from build123d import *

# Parameters (mm, degrees)
SKETCH1_W           = 70
SKETCH1_H           = 170
BOSS_EXTRUDE1_DEPTH = 5
SKETCH2_W           = 70
SKETCH2_H           = 5
BOSS_EXTRUDE2_DEPTH = 25
SKETCH3_W           = 70
SKETCH3_H           = 5
BOSS_EXTRUDE3_DEPTH = 50
SKETCH4_W           = 3
SKETCH4_H           = 15
BOSS_EXTRUDE4_DEPTH = 20
CUT_EXTRUDE1_REACH  = 98.695
SKETCH6_R           = 12.5
SKETCH6_R_2         = 7
SKETCH6_R_3         = 8.5
SKETCH6_R_4         = 8
SKETCH6_R_5         = 4.5
SKETCH6_R_6         = 3
SKETCH7_R           = 4.797792648
SKETCH7_R_2         = 3.987535838
SKETCH7_W           = 10.549301712
SKETCH7_H           = 5.014130384
BOSS_EXTRUDE5_DEPTH = 3


with BuildPart() as part:
    # Sketch1 → Boss-Extrude1 (new body)
    with BuildSketch(Plane.XY):
        Rectangle(SKETCH1_W, SKETCH1_H)
    extrude(amount=BOSS_EXTRUDE1_DEPTH)

    # Sketch2 → Boss-Extrude2 (add)
    with BuildSketch(Plane.XY.offset(5)):
        with Locations((0, -82.5)):
            Rectangle(SKETCH2_W, SKETCH2_H)
    extrude(amount=BOSS_EXTRUDE2_DEPTH)

    # Sketch3 → Boss-Extrude3 (add)
    with BuildSketch(Plane(origin=(0, -80, 0), x_dir=(1, 0, 0), z_dir=(0, 1, 0))):
        with Locations((0, -27.5)):
            Rectangle(SKETCH3_W, SKETCH3_H)
    extrude(amount=BOSS_EXTRUDE3_DEPTH)

    # Sketch4 → Boss-Extrude4 (add)
    with BuildSketch(Plane.XY.offset(5)):
        with Locations((-33.5, -37.5)):
            Rectangle(SKETCH4_W, SKETCH4_H)
        with Locations((33.5, -37.5)):
            Rectangle(SKETCH4_W, SKETCH4_H)
    extrude(amount=BOSS_EXTRUDE4_DEPTH)

    # Sketch6 → Cut-Extrude1 (cut, up to next)
    with BuildSketch(Plane.XY.offset(30), mode=Mode.PRIVATE) as cut_extrude1_sk1:
        with Locations((0, -45)):
            Circle(SKETCH6_R)
    cut_extrude1_tool1 = extrude(cut_extrude1_sk1.sketch, amount=-CUT_EXTRUDE1_REACH, mode=Mode.PRIVATE) & part.part
    # Sketch6 → Cut-Extrude1 (cut, up to next)
    with BuildSketch(Plane.XY.offset(30), mode=Mode.PRIVATE) as cut_extrude1_sk2:
        with Locations((-25, -40)):
            Circle(SKETCH6_R_2)
    cut_extrude1_tool2 = extrude(cut_extrude1_sk2.sketch, amount=-CUT_EXTRUDE1_REACH, mode=Mode.PRIVATE) & part.part
    # Sketch6 → Cut-Extrude1 (cut, up to next)
    with BuildSketch(Plane.XY.offset(30), mode=Mode.PRIVATE) as cut_extrude1_sk3:
        with Locations((25, -40)):
            Circle(SKETCH6_R_2)
    cut_extrude1_tool3 = extrude(cut_extrude1_sk3.sketch, amount=-CUT_EXTRUDE1_REACH, mode=Mode.PRIVATE) & part.part
    # Sketch6 → Cut-Extrude1 (cut, up to next)
    with BuildSketch(Plane.XY.offset(30), mode=Mode.PRIVATE) as cut_extrude1_sk4:
        with Locations((-20, -60)):
            Circle(SKETCH6_R_3)
    cut_extrude1_tool4 = extrude(cut_extrude1_sk4.sketch, amount=-CUT_EXTRUDE1_REACH, mode=Mode.PRIVATE) & part.part
    # Sketch6 → Cut-Extrude1 (cut, up to next)
    with BuildSketch(Plane.XY.offset(30), mode=Mode.PRIVATE) as cut_extrude1_sk5:
        with Locations((20, -60)):
            Circle(SKETCH6_R_3)
    cut_extrude1_tool5 = extrude(cut_extrude1_sk5.sketch, amount=-CUT_EXTRUDE1_REACH, mode=Mode.PRIVATE) & part.part
    # Sketch6 → Cut-Extrude1 (cut, up to next)
    with BuildSketch(Plane.XY.offset(30), mode=Mode.PRIVATE) as cut_extrude1_sk6:
        with Locations((0, -70)):
            Circle(SKETCH6_R_4)
    cut_extrude1_tool6 = extrude(cut_extrude1_sk6.sketch, amount=-CUT_EXTRUDE1_REACH, mode=Mode.PRIVATE) & part.part
    # Sketch6 → Cut-Extrude1 (cut, up to next)
    with BuildSketch(Plane.XY.offset(30), mode=Mode.PRIVATE) as cut_extrude1_sk7:
        with Locations((-17, -75)):
            Circle(SKETCH6_R_5)
    cut_extrude1_tool7 = extrude(cut_extrude1_sk7.sketch, amount=-CUT_EXTRUDE1_REACH, mode=Mode.PRIVATE) & part.part
    # Sketch6 → Cut-Extrude1 (cut, up to next)
    with BuildSketch(Plane.XY.offset(30), mode=Mode.PRIVATE) as cut_extrude1_sk8:
        with Locations((17, -75)):
            Circle(SKETCH6_R_5)
    cut_extrude1_tool8 = extrude(cut_extrude1_sk8.sketch, amount=-CUT_EXTRUDE1_REACH, mode=Mode.PRIVATE) & part.part
    # Sketch6 → Cut-Extrude1 (cut, up to next)
    with BuildSketch(Plane.XY.offset(30), mode=Mode.PRIVATE) as cut_extrude1_sk9:
        with Locations((29, -75)):
            Circle(SKETCH6_R_6)
    cut_extrude1_tool9 = extrude(cut_extrude1_sk9.sketch, amount=-CUT_EXTRUDE1_REACH, mode=Mode.PRIVATE) & part.part
    # Sketch6 → Cut-Extrude1 (cut, up to next)
    with BuildSketch(Plane.XY.offset(30), mode=Mode.PRIVATE) as cut_extrude1_sk10:
        with Locations((-29, -75)):
            Circle(SKETCH6_R_6)
    cut_extrude1_tool10 = extrude(cut_extrude1_sk10.sketch, amount=-CUT_EXTRUDE1_REACH, mode=Mode.PRIVATE) & part.part
    add(cut_extrude1_tool1.solids().sort_by_distance((0, -45, 30))[0], mode=Mode.SUBTRACT)
    add(cut_extrude1_tool2.solids().sort_by_distance((-25, -40, 30))[0], mode=Mode.SUBTRACT)
    add(cut_extrude1_tool3.solids().sort_by_distance((25, -40, 30))[0], mode=Mode.SUBTRACT)
    add(cut_extrude1_tool4.solids().sort_by_distance((-20, -60, 30))[0], mode=Mode.SUBTRACT)
    add(cut_extrude1_tool5.solids().sort_by_distance((20, -60, 30))[0], mode=Mode.SUBTRACT)
    add(cut_extrude1_tool6.solids().sort_by_distance((0, -70, 30))[0], mode=Mode.SUBTRACT)
    add(cut_extrude1_tool7.solids().sort_by_distance((-17, -75, 30))[0], mode=Mode.SUBTRACT)
    add(cut_extrude1_tool8.solids().sort_by_distance((17, -75, 30))[0], mode=Mode.SUBTRACT)
    add(cut_extrude1_tool9.solids().sort_by_distance((29, -75, 30))[0], mode=Mode.SUBTRACT)
    add(cut_extrude1_tool10.solids().sort_by_distance((-29, -75, 30))[0], mode=Mode.SUBTRACT)

    # Sketch7 → Boss-Extrude5 (add)
    with BuildSketch(Plane.XY.offset(5)):
        with Locations((-19.294668455, -21.257959738)):
            Circle(SKETCH7_R)
        with Locations((19.294668455, -21.257959738)):
            Circle(SKETCH7_R_2)
        with Locations((-29.725349144, 82.492934808)):
            Rectangle(SKETCH7_W, SKETCH7_H)
        with Locations((29.725349144, 82.492934808)):
            Rectangle(SKETCH7_W, SKETCH7_H)
    extrude(amount=BOSS_EXTRUDE5_DEPTH)


solid = part.part
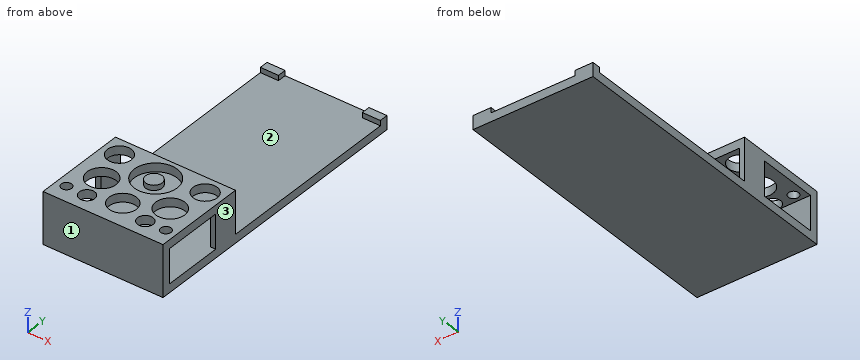
Part model, mm, in its own coordinate system. Face numbers are marked on the shaded views. Coordinates: 2 decimals unless noted, no trailing zeros. Write each loop counter-clockwise with the first axis right and the second up, starting at its lowest first coordinate (ties: lowest second). Pieces come first, ordered by that corner, then holes. Notation, with made-up numbers: (17, 61.25) - (47, 61.25) arc R24 cw to (47, 72.25) - close; hole circle Ø5 at (73, 79). An arc over 180 degrees is marked (long way). Put each result on its own line as item: value.
1. Two-plate mould, pull along Y, no slides. Class the marked faces 1, 2 and 3: +Y half, -Y half, draft (parallel to the pull), parting line (faces both ways), or undercut.
Final values:
face 1: -Y half
face 2: undercut
face 3: draft
2. Band-saw the part on A-A (y = -60). Write the cut outline in (x, z), then the cut area to 3 significant figures.
Final values:
outline: (-35, 0) - (35, 0) - (35, 5) - (-35, 5) - close; (-35, 25) - (-28.5, 25) - (-28.5, 30) - (-35, 30) - close; (-11.5, 25) - (11.5, 25) - (11.5, 30) - (-11.5, 30) - close; (28.5, 25) - (35, 25) - (35, 30) - (28.5, 30) - close
area: 530 mm²
3. Flat gauge pins, fed straight in: pin 1 Ø2 at (x, y) = (17, 51) entering from -Z; pin 2 Ø6 at (y, z) = (-15.5, 9.5) entering from -X; pin 3 Ø1.5 at (x, y) = (-29.5, 83) entering from +Z. Where does each tip first touch, or does it go through?
Final values:
pin 1: stops at z = 0
pin 2: stops at x = -22.9
pin 3: stops at z = 8
4. Band-saw the part on B-B (x = 0). Write the cut outline in (y, z).
Final values:
outline: (-85, 0) - (85, 0) - (85, 5) - (-80, 5) - (-80, 25) - (-78, 25) - (-78, 30) - (-85, 30) - close; (-62, 25) - (-57.5, 25) - (-57.5, 30) - (-62, 30) - close; (-32.5, 25) - (-30, 25) - (-30, 30) - (-32.5, 30) - close
5. Band-saw the part on C-C (z = 27). Give the number of separate pieces and of enclosed holes in the cut face, then the cut area to 3 significant figures.
Final values:
separate pieces: 1
enclosed holes: 10
area: 2,210 mm²
6. Probe line 1 along Y through (x, z) = (29, 28.85); line 2 along Y through (x, z) = (0, 28.7); line 3 along Z through (x, y) = (-8.5, 43). List the from-to ranges inside material, lowest first. Write a range as [from, to].
Final values:
line 1: y = [-85, -78], [-72, -45.74], [-34.26, -30]
line 2: y = [-85, -78], [-62, -57.5], [-32.5, -30]
line 3: z = [0, 5]
7. Band-saw the part on D-D (z = 9.5). Write the cut outline in (x, y), then the cut area to 3 significant figures.
Final values:
outline: (-35, -85) - (35, -85) - (35, -80) - (-35, -80) - close; (-35, -45) - (-32, -45) - (-32, -30) - (-35, -30) - close; (32, -45) - (35, -45) - (35, -30) - (32, -30) - close
area: 440 mm²
